Work out the finished part from the listing and answer in its coordinate system (mm). A direction names the side the tool comes from. Round coordinates to 2 decimals unless told otherwise and drop trailing zeros. Order: outer loops, then holes, each group sorted by start corner. A loop starts at its lowest first (then second) coordinate and runs counter-clockwise, first axis right, second up. Notation, with made-up numbers: (83, 26.5) - (93, 26.5) arc R23 cw to (93, 37.5) - close; hole circle Ø7 at (-33.5, 80). An arc over 180 degrees is marked (long way). Use one line per item in the form item = value. Start each with the question number.
Q1. The part is cut by section C-C on x = 3.75. Determine the outline of the cut face in (y, z), plus the area to 3 significant figures.
Q2. For a pull along Y with two mould halves and no side action, classify faces 1 (the cylindrical face through (1.01, 5.37, -1.19)), 2 (the flat face through (6.1, 1, 4)), 3 (the flat face through (18, 0, -4)) as +Y half, -Y half, draft (parallel to the pull), parting line (faces both ways), or undercut.
Q3. The part is cut by section D-D on z = 4. Determine the outline of the cut face in (x, y).
Q4. Given P1, Ø3, axis at x = 9, z = -4, coming from the +Y side; P2, Ø5.5, axis at y = -1.5, z = 0.5, coming from the +X side; P3, Ø4, axis at x = 12.5, z = -3, coming from the -Y side; P4, Ø2.5, axis at x = 15.2, y = 0, coming from the +Z side, each flat-ended and moving along its own axis, determine where each tip first touches the part or whether it passes through.
Q5. Which of the six approach directions +Z, -Z, +X, -X, +Y, -Y give full straight-line access (tool end or side, diameter ignored) to faces 4 (the cylindrical face through (13.736, -1.52, 4.826)), 5 (the cylindrical face through (3.007, 4.637, -1.03)), 6 (the cylindrical face through (2.608, -1.569, 4.984))?
Q6. The part is cut by section A-A on y = 0. State how many separate pieces and enclosed holes the cut face has, plus the area to 3 significant figures.
Q7. The part is cut by section B-B on z = 0. Determine the outline of the cut face in (x, y) (3 decimals), plus the area to 3 significant figures.
Q8. Find the intervals of material crossed by line 1 (Y direction, x = 13, z = 0); line 2 (X direction, y = 0, z = -4.5); line 3 (Y direction, x = 4.5, z = 0), in increasing order. Write a range as [from, to].
from build123d import *

# Parameters (mm, degrees)
ESBO_O2_R             = 1
CORTE_EXTRUS_O1_DEPTH = 10


with BuildPart() as part:
    # Esboço1 → Revolução1 (revolve)
    with BuildSketch(Plane.XY, mode=Mode.PRIVATE) as revolu_o1_sk:
        Polygon((0, 5.5), (2, 5.5), (2, 5.225), (3.2, 5.225), (3.2, 5.5), (9.35, 5.5), (9.35, 5.06), (18, 5.06), (18, 3.75), (6.1, 3.75), (6.1, 4.75), (0, 4.75), align=None)
    revolve(revolu_o1_sk.sketch.rotate(Axis((0, 0, 0), (1, 0, 0)), 90), axis=Axis((0, 0, 0), (1, 0, 0)))

    # Esboço2 → Corte-extrusão1 (cut, symmetric)
    with BuildSketch(Plane.XY):
        with Locations((15.2, 0)):
            Circle(ESBO_O2_R)
    extrude(amount=CORTE_EXTRUS_O1_DEPTH, both=True, mode=Mode.SUBTRACT)


solid = part.part
Found:
q1.outline = circle Ø11 at (0, 0); hole circle Ø9.5 at (0, 0)
q1.area = 24.2 mm²
q2.face_1 = parting line
q2.face_2 = undercut
q2.face_3 = draft
q3.outline = (0, -3.77) - (2, -3.77) - (2, -3.36) - (3.2, -3.36) - (3.2, -3.77) - (9.35, -3.77) - (9.35, -3.1) - (18, -3.1) - (18, 3.1) - (9.35, 3.1) - (9.35, 3.77) - (3.2, 3.77) - (3.2, 3.36) - (2, 3.36) - (2, 3.77) - (0, 3.77) - (0, 2.56) - (6.1, 2.56) - (6.1, -2.56) - (0, -2.56) - close; hole circle Ø2 at (15.2, 0)
q4.P1 = 4.9
q4.P2 = 18
q4.P3 = -4.96
q4.P4 = 5.06
q5.face_4 = +X
q5.face_5 = -X
q5.face_6 = none
q6.separate_pieces = 4
q6.enclosed_holes = 0
q6.area = 37.3 mm²
q7.outline = (0, -5.5) - (2, -5.5) - (2, -5.225) - (3.2, -5.225) - (3.2, -5.5) - (9.35, -5.5) - (9.35, -5.06) - (18, -5.06) - (18, -3.75) - (6.1, -3.75) - (6.1, -4.75) - (0, -4.75) - close; (0, 4.75) - (6.1, 4.75) - (6.1, 3.75) - (18, 3.75) - (18, 5.06) - (9.35, 5.06) - (9.35, 5.5) - (3.2, 5.5) - (3.2, 5.225) - (2, 5.225) - (2, 5.5) - (0, 5.5) - close
q7.area = 42.5 mm²
q8.line_1 = [-5.06, -3.75], [3.75, 5.06]
q8.line_2 = [6.1, 14.2], [16.2, 18]
q8.line_3 = [-5.5, -4.75], [4.75, 5.5]
